Check sheet for the modelled part. Datum: model origin and axes. Units: mm. Coordinates: 2 decimals unless noted, no trailing zeros. Write each loop counter-clockwise with the first axis right and the second up, starting at its lowest first coordinate (ties: lowest second). Pieces come first, ordered by that corner, then holes. Notation, with made-up numbers: (-11, 78) -> (42, 78) arc R26 cw to (42, 92) -> close; hole circle Ø6 at (35.5, -4). An arc over 180 degrees is marked (long way). Put each result on its own line as item: value.
```python
from build123d import *

# Parameters (mm, degrees)
SKETCH_1_R      = 1.65
SKETCH_1_R_2    = 1
EXTRUDE_1_DEPTH = 2


with BuildPart() as part:
    # Эскиз1 → Бобышка-Вытянуть1 (new body)
    with BuildSketch(Plane(origin=(0, 0, 0), x_dir=(1, 0, 0), z_dir=(0, 1, 0))):
        with BuildLine():
            Line((0, 10), (80, 10))
            ThreePointArc((80, 10), (90, 0), (80, -10))
            Line((80, -10), (0, -10))
            ThreePointArc((0, -10), (-10, 0), (0, 10))
        make_face()
        with Locations(Location((30, 0, 0), (0, 0, 270))):
            Circle(SKETCH_1_R, mode=Mode.SUBTRACT)
        with Locations(Location((0, 0, 0), (0, 0, 270))):
            Circle(SKETCH_1_R, mode=Mode.SUBTRACT)
        with Locations(Location((15, 0, 0), (0, 0, 270))):
            Circle(SKETCH_1_R, mode=Mode.SUBTRACT)
        with Locations(Location((80, 7, 0), (0, 0, 270))):
            Circle(SKETCH_1_R_2, mode=Mode.SUBTRACT)
        with Locations(Location((87, 0, 0), (0, 0, 270))):
            Circle(SKETCH_1_R_2, mode=Mode.SUBTRACT)
        with Locations(Location((73, 0, 0), (0, 0, 270))):
            Circle(SKETCH_1_R_2, mode=Mode.SUBTRACT)
        with Locations(Location((80, -7, 0), (0, 0, 270))):
            Circle(SKETCH_1_R_2, mode=Mode.SUBTRACT)
    extrude(amount=EXTRUDE_1_DEPTH)


solid = part.part
```
Q1. Depth check by flat-ended pin: P1, Ø2.5, axis at x = 30, z = 0, coming from the +Y side. Enter the tip coordinate at first touch or a pass-through.
Recorded:
P1: passes through
Q2. Cross-section at A-A (x = 73). Record the cut outline in (y, z), plus the area to 3 significant figures.
Recorded:
outline: (0, -10) -> (2, -10) -> (2, -1) -> (0, -1) -> close; (0, 1) -> (2, 1) -> (2, 10) -> (0, 10) -> close
area: 36.0 mm2
Q3. Mould release check, pull along X, two halves, no side actions. Record for faces 1 (the flat face through (41, 2, 0)), 2 (the cylindrical face through (-1, 0.99, -1.31)), 3 (the cylindrical face through (-10, 1, 0)): released by +X, released by -X, zero draft, split by the parting line, or undercut.
Recorded:
face 1: zero draft
face 2: undercut
face 3: released by -X
Q4. Material ranges on line 1 along Z through (x, y) = (80, 1.45); line 2 along X through (y, z) = (0.85, 0); line 3 along X through (y, z) = (1.8, 1.25), recorded low to high.
Recorded:
line 1: z = -10 to -8, -6 to 6, 8 to 10
line 2: x = -10 to -1.65, 1.65 to 13.35, 16.65 to 28.35, 31.65 to 72, 74 to 86, 88 to 90
line 3: x = -9.92 to -1.08, 1.08 to 13.92, 16.08 to 28.92, 31.08 to 89.92
Q5. Cross-section at C-C (y = 0.3). Record the cut outline in (x, z).
Recorded:
outline: (0, -10) -> (80, -10) arc R10 ccw to (80, 10) -> (0, 10) arc R10 ccw to start; hole circle Ø3.3 at (0, 0); hole circle Ø3.3 at (15, 0); hole circle Ø3.3 at (30, 0); hole circle Ø2 at (73, 0); hole circle Ø2 at (80, -7); hole circle Ø2 at (80, 7); hole circle Ø2 at (87, 0)
Q6. Cross-section at B-B (z = 0). Record the cut outline in (x, y), plus the area to 3 significant figures.
Recorded:
outline: (-10, 0) -> (-1.65, 0) -> (-1.65, 2) -> (-10, 2) -> close; (1.65, 0) -> (13.35, 0) -> (13.35, 2) -> (1.65, 2) -> close; (16.65, 0) -> (28.35, 0) -> (28.35, 2) -> (16.65, 2) -> close; (31.65, 0) -> (72, 0) -> (72, 2) -> (31.65, 2) -> close; (74, 0) -> (86, 0) -> (86, 2) -> (74, 2) -> close; (88, 0) -> (90, 0) -> (90, 2) -> (88, 2) -> close
area: 172 mm2
Q7. Cross-section at D-D (z = 7). Record the cut outline in (x, y), plus the area to 3 significant figures.
Recorded:
outline: (-7.14, 0) -> (79, 0) -> (79, 2) -> (-7.14, 2) -> close; (81, 0) -> (87.14, 0) -> (87.14, 2) -> (81, 2) -> close
area: 185 mm2
